Design review of the part built by this model. Coordinates are the model's own, in mm. A direction names the side the tool comes from. Coordinates: 2 decimals unless noted, no trailing zeros. Order: outer loops, then holes, each group sorted by start corner. A loop starts at its lowest first (then second) coordinate and runs counter-clockwise, first axis right, second up. Notation, with made-up numbers: M 11,19.25 L 59,19.25 A15 cw 59,39.25 Z; hole C 43,-1.5 d2. An arc over 180 degrees is marked long. Use CSV: the item, a comma, the result in double quotes.
```python
from build123d import *

# Parameters (mm, degrees)
SKETCH2_R           = 17.4625
BOSS_EXTRUDE1_DEPTH = 18
SKETCH13_R          = 0.8
CUT_EXTRUDE6_DEPTH  = 10
SKETCH16_R          = 11
CUT_EXTRUDE9_DEPTH  = 15
CUT_EXTRUDE11_DEPTH = 22
SKETCH21_W          = 16.25
SKETCH21_H          = 2.78436417
CUT_EXTRUDE12_DEPTH = 31.559414466
CUT_EXTRUDE13_REACH = 32.559
SKETCH24_W          = 16.25
SKETCH24_H          = 6.70136321
CUT_EXTRUDE14_DEPTH = 17


with BuildPart() as part:
    # Sketch2 → Boss-Extrude1 (new body)
    with BuildSketch(Plane.XY):
        Circle(SKETCH2_R)
    extrude(amount=BOSS_EXTRUDE1_DEPTH)

    # Sketch13 → Cut-Extrude6 (cut)
    with BuildSketch(Plane.XY.offset(18)):
        with Locations((0, 13.5)):
            Circle(SKETCH13_R)
        with Locations((11.691342951, -6.75)):
            Circle(SKETCH13_R)
        with Locations((-11.691342951, -6.75)):
            Circle(SKETCH13_R)
    extrude(amount=-CUT_EXTRUDE6_DEPTH, mode=Mode.SUBTRACT)

    # Sketch16 → Cut-Extrude9 (cut)
    with BuildSketch(Plane.XY.offset(18)):
        Circle(SKETCH16_R)
    extrude(amount=-CUT_EXTRUDE9_DEPTH, mode=Mode.SUBTRACT)

    # Sketch20 → Cut-Extrude11 (cut)
    with BuildSketch(Plane(origin=(5.95728493, 0, -11.08430825), x_dir=(0, 0, 1), z_dir=(0, 1, 0))):
        Polygon((16.52930825, -11.021800725), (16.52930825, -6.906800725), (14.92930825, -6.906800725), (14.92930825, -4.926800725), (16.52930825, -4.926800725), (16.52930825, -0.811800725), (18.05430825, -0.811800725), (18.05430825, 1.028199275), (22.11430825, 1.028199275), (22.11430825, -0.811800725), (23.63930825, -0.811800725), (23.63930825, -11.021800725), (22.11430825, -11.021800725), (22.11430825, -12.861800725), (18.05430825, -12.861800725), (18.05430825, -11.021800725), align=None)
    extrude(amount=-CUT_EXTRUDE11_DEPTH, mode=Mode.SUBTRACT)

    # Sketch21 → Cut-Extrude12 (cut, through all)
    with BuildSketch(Plane.XY.offset(18)):
        with Locations((0, -16.852182085)):
            Rectangle(SKETCH21_W, SKETCH21_H)
    extrude(amount=-CUT_EXTRUDE12_DEPTH, mode=Mode.SUBTRACT)

    # Cut-Extrude13: up to this face of the body (flat: up to its plane)
    cut_extrude13_end = Plane(part.part.faces().sort_by_distance((0, 0, 3))[0])
    # Sketch24 → Cut-Extrude13 (cut, up to the picked face)
    with BuildSketch(Plane.XY.offset(18), mode=Mode.PRIVATE) as cut_extrude13_sk1:
        with Locations((0.005436819, -10.109318395)):
            Rectangle(SKETCH24_W, SKETCH24_H)
    cut_extrude13_tool1 = split(extrude(cut_extrude13_sk1.sketch, amount=-CUT_EXTRUDE13_REACH, mode=Mode.PRIVATE), bisect_by=cut_extrude13_end, keep=Keep.BOTH, mode=Mode.PRIVATE)
    add(cut_extrude13_tool1.solids().sort_by(Axis((0.005437, -10.109318, 18), (0, 0, -1)))[0], mode=Mode.SUBTRACT)

    # Sketch26 → Cut-Extrude14 (cut)
    with BuildSketch(Plane.XY.offset(18)):
        Polygon((-8.119563181, -14.21), (-8.119563181, -15.46), (8.119563181, -15.46), (8.119563181, -14.21), (8.890436819, -14.21), (8.890436819, -13.46), (8.130436819, -13.46), (-8.119563181, -13.46), (-8.879563181, -13.46), (-8.879563181, -14.21), align=None)
    extrude(amount=-CUT_EXTRUDE14_DEPTH, mode=Mode.SUBTRACT)


solid = part.part
```
(1) Add section A-A on x = 0. State the section outline as (y, z) points, and give its area (3 significant figures).
The answers:
outline,"M -15.46,0 L 17.46,0 L 17.46,18 L 14.3,18 L 14.3,8 L 12.7,8 L 12.7,18 L 11,18 L 11,3 L -13.46,3 L -13.46,1 L -15.46,1 Z"
area,"176 mm2"
(2) Wall thickness on probe 1 along Y at (x, z) = (0, 10.5); probe 2 along X at (y, z) = (0, 10.75); probe 3 along X at (y, z) = (-7, 14.75): over which ranges is each line inside the solid? List them lowest first.
The answers:
probe 1,"y = 11 to 12.7, 14.3 to 17.46"
probe 2,"x = -17.46 to -11, 11 to 17.46"
probe 3,"x = -16 to -12.45, -10.93 to -8.49, 8.49 to 10.93, 12.45 to 16"
(3) Add section C-C on y = 0. State the section outline as (x, z) points.
The answers:
outline,"M -17.46,0 L 17.46,0 L 17.46,18 L 11,18 L 11,3 L -11,3 L -11,18 L -17.46,18 Z"
(4) For faces 4 (the face through (-12, -7, 8)), 5 (the face through (0, 1, 0)), 6 (the face through (-8.12, -10, 11)), list the 3-axis set-ups (+Z, -Z, +X, -X, +Y, -Y) from which the entire face can be reached by the end or side of a thin tool; tool diameter is ignored.
The answers:
face 4,"+Z"
face 5,"-Z, +X, -X, +Y, -Y"
face 6,"+Z, -Y"
(5) Clearance check with flat-ended pins moving along their axes: P1, Ø6, axis at x = -7, z = 11.5, coming from the +Y side; P2, Ø1.3, axis at x = 11.69, y = -6.75, coming from the +Z side; P3, Ø6, axis at y = 12, z = 9, coming from the +X side. State where each tip first meets the part, or that it passes through.
The answers:
P1,"stops at y = 17"
P2,"stops at z = 8"
P3,"stops at x = 14.96"
(6) Add section D-D on z = 14.5. Give the number of separate pieces and of enclosed holes in the cut face, and give its area (3 significant figures).
The answers:
separate pieces,"1"
enclosed holes,"3"
area,"458 mm2"
(7) The part is to be moulded in two halves that separate along Y. For faces 1 (the face through (8.12, -15, 10)), 2 (the face through (-1.3, -13.46, 2.6)), 3 (the face through (0.65, 17.45, 8.87)), say which applies: pulls with the +Y half, pulls with the -Y half, needs draft (parallel to the pull), parting line crosses it, or undercut.
The answers:
face 1,"needs draft"
face 2,"undercut"
face 3,"parting line crosses it"
(8) Add section B-B on z = 4. State the section outline as (x, y) points (1 decimal).
The answers:
outline,"M -8.9,-14.2 L -8.9,-13.5 L -8.1,-13.5 L -8.1,-7.4 A11 cw long 8.1,-7.4 L 8.1,-13.5 L 8.9,-13.5 L 8.9,-14.2 L 8.1,-14.2 L 8.1,-15.5 A17.5 ccw long -8.1,-15.5 L -8.1,-14.2 Z"
